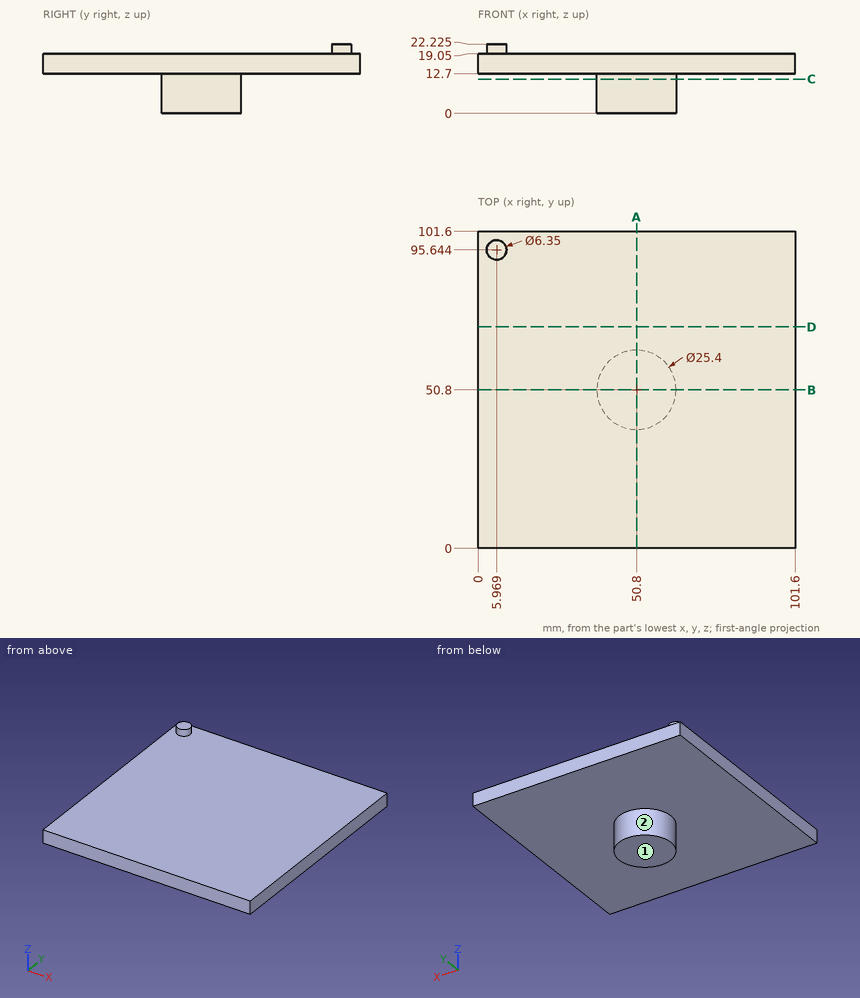
Geometry: see drawing. Coordinates: mm, zero at the bounding-box minimum. A direction names the side the tool comes from. Coordinates: 2 decimals unless noted, no trailing zeros. Loops run counter-clockwise (first coordinate to the right, second up) from the corner with the lowest first, then second, coordinate; pieces in that order, holes last.
(1) Material intervals for probe 1 along Z at (x, y) = (65, 80); probe 2 along Z at (x, y) = (51, 61.5), sorted ascending.
(2) Section D-D on y = 71. Return the cut outline in (x, z).
(3) First-contact query: pin 1 Ø6 at (x, y) = (30, 47.5) entering from +Z. Flat tip, straight axial feed; report the tip coordinate or a pass-through.
(4) Set-up query: the marked faces 1 and 2. Return all of +Z, -Z, +X, -X, +Y, -Y with unobstructed straight access to the full face (end or side cutting, diameter ignored); none if empty.
(5) Section A-A on x = 50.8. Return the cut outline in (y, z), then the cut area to 3 significant figures.
(6) Section C-C on z = 11. Return the cut outline in (x, y).
Data:
1. probe 1: z = 12.7 to 19.05
1. probe 2: z = 0 to 19.05
2. outline: (0, 12.7) - (101.6, 12.7) - (101.6, 19.05) - (0, 19.05) - close
3. pin 1: stops at z = 19.05
4. face 1: -Z, +X, -X, +Y, -Y
4. face 2: -Z
5. outline: (0, 12.7) - (38.1, 12.7) - (38.1, 0) - (63.5, 0) - (63.5, 12.7) - (101.6, 12.7) - (101.6, 19.05) - (0, 19.05) - close
5. area: 968 mm2
6. outline: circle Ø25.4 at (50.8, 50.8)
